Autodesk Inventor part; units mm, degrees
ref_plane "YZ Plane" through (0, 0, 0) normal (1, 0, 0) x (0, 1, 0)
ref_plane "XZ Plane" through (0, 0, 0) normal (0, 1, 0) x (-1, 0, 0)
ref_plane "XY Plane" through (0, 0, 0) normal (0, 0, 1) x (1, 0, 0)
sketch "Sketch1" plane through (0, 0, 0) normal (0, 1, 0) x (-1, 0, 0)
  arc A0 (0, -50) -> (0, 0) centre (-48.9898, -25) ccw
  arc A1 (0, -49) -> (0, -1) centre (-49.4874, -25) ccw
  line L0 (0, 0) -> (0, -50)
  line L1 (0, -12.5) -> (5.5721, -18.0721)
  line L2 (0, -12.5) -> (7.8802, -12.5) construction
  line L3 (0, -13.5) -> (5.704, -19.204)
  line L4 (0, -25) -> (5.7127, -30.7127)
  line L5 (0, -25) -> (8.079, -25) construction
  line L6 (0, -26) -> (5.6114, -31.6114)
  line L7 (0, -35) -> (4.157, -39.157)
  line L8 (0, -35) -> (5.8789, -35) construction
  line L9 (0, -36) -> (3.9417, -39.9417)
  arc A2 (0, 0) -> (0, -50) centre (48.9898, -25) ccw
  arc A3 (0, -1) -> (0, -49) centre (49.4874, -25) ccw
  line L10 (0, -12.5) -> (-5.5721, -18.0721)
  line L11 (0, -13.5) -> (-5.704, -19.204)
  line L12 (0, -25) -> (-5.7127, -30.7127)
  line L13 (0, -26) -> (-5.6114, -31.6114)
  line L14 (0, -35) -> (-4.157, -39.157)
  line L15 (0, -36) -> (-3.9417, -39.9417)
  line L16 (0.5, 0) -> (0.5, -50.0047)
  line L17 (-0.5, 0) -> (-0.5, -50.0047)
  point P0 (5.1659, -31.1659)
  point P1 (3.7628, -38.7628)
  point P2 (0.5, -35.5)
  point P3 (0.5, -26.5)
  point P4 (-3.7628, -38.7628)
  point P5 (-5.1659, -31.1659)
  point P6 (-0.5, -26.5)
  point P7 (-0.5, -35.5)
  point P8 (-5.2605, -30.2605)
  point P9 (-5.1441, -18.6441)
  point P10 (-0.5, -14)
  point P11 (-0.5, -25.5)
  point P12 (-4.9987, -17.4987)
  point P13 (-0.5, -2.0596)
  point P14 (-0.5, -13)
  point P15 (-0.5, -36.5)
  point P16 (-0.5, -47.9404)
  point P17 (-3.5525, -39.5525)
  point P18 (4.9987, -17.4987)
  point P19 (0.5, -13)
  point P20 (0.5, -2.0596)
  point P21 (3.5525, -39.5525)
  point P22 (0.5, -47.9404)
  point P23 (0.5, -36.5)
  point P24 (5.1441, -18.6441)
  point P25 (5.2605, -30.2605)
  point P26 (0.5, -25.5)
  point P27 (0.5, -14)
  dimension "d0" = 50
  dimension "d1" = 55
  dimension "d2" = 48
  dimension "d3" = 55
  dimension "d4" = 45
  dimension "d5" = 45
  dimension "d6" = 45
extrude "Extrusion1" add sketch "Sketch1" along normal blind 20 contours L9 A1 L7 A0 | A0 L16 A1 L9 | L7 A1 L6 A0 | A0 L0 A1 L16 | L9 L16 L7 A1 | L6 A1 L4 A0 | A2 L17 A3 L0 | A1 L0 L9 L16 | L9 L0 L7 L16 | L4 A1 L3 A0 | L6 L16 L4 A1 | L7 L0 L6 L16 | A3 L17 L15 L0 | A2 L15 A3 L17 | L15 L17 L14 L0 | L3 A1 L1 A0 | L6 L0 L4 L16 | L14 L17 L13 L0 | A2 L14 A3 L15 | L15 A3 L14 L17 | L1 A1 L16 A0 | L3 L16 L1 A1 | L4 L0 L3 L16 | L13 L17 L12 L0 | A2 L13 A3 L14 | L16 A1 L0 A0 | L3 L0 L1 L16 | L12 L17 L11 L0 | L13 A3 L12 L17 | A2 L12 A3 L13 | L0 A3 L17 A2 | L16 L1 L0 A1 | L11 L17 L10 L0 | A2 L11 A3 L12 | L0 L10 L17 A3 | L17 A3 L10 A2 | L11 A3 L10 L17 | A2 L10 A3 L11
sketch "Sketch2" plane through (0, 0, 0) normal (0, 0, 1) x (1, 0, 0)
  point P0 (0, 0)
sketch "Sketch3" plane through (0, 0, 0) normal (1, 0, 0) x (0, 1, 0)
  line L0 (0, 0) -> (20, 0)
  line L1 (0, -50) -> (20, -50)
  arc A0 (10, 0) -> (10, -50) centre (64.5436, -25) ccw
  arc A1 (11, 0) -> (11, -50) centre (65.5436, -25) ccw
  line L2 (11, 0) -> (11, -50) construction
  line L3 (11, 0) -> (61, 0) construction
  line L4 (11, 0) -> (20, 0)
  line L5 (20, -50) -> (20, 0)
  line L6 (20, 0) -> (20, -50)
  line L7 (20, -50) -> (11, -50)
  line L8 (10, 0) -> (0, 0)
  line L9 (0, 0) -> (0, -50)
  line L10 (10, -50) -> (0, -50)
  point P0 (11, 0)
  point P1 (11, -50)
  dimension "d9" = 60
  dimension "d10" = 50
  dimension "d11" = 90
  dimension "d12" = 60
extrude "Extrusion2" cut sketch "Sketch3" along normal mid plane 20 contours L0 A0 L1 L9 | L0 L5 L1 A1
Check sheet for the modelled part. Datum: model origin and axes. Units: mm. Give positions to 0.01 mm unless a question says otherwise; leave off trailing zeros. Order: outer loops, then holes, each group sorted by start corner. A loop starts at its lowest first (then second) coordinate and runs counter-clockwise, first axis right, second up. Notation, with made-up numbers: M 43.25,33 L 73.25,33 A25 ccw 73.25,68 Z; hole C -0.5,45 d11. An arc over 180 degrees is marked long. Answer as CSV lines item,"result". Start each with the question number.
Item 1: Cross-section at C-C on y = 7.75. Enter the section's corners in (x, z).
Item 2: Cross-section at B-B on x = -1.75. Enter the section's corners in (y, z).
Item 3: Thickness scan on line 1 (X direction, y = 6, z = -33.5); line 2 (Z direction, x = -0.75, y = 9.75); line 3 (Z direction, x = 3.5, y = 5.5). Record the ranges inside material, lowest first. Write a range as [from, to].
Item 4: Cross-section at D-D on x = -4.5. Enter the section's corners in (y, z).
Item 5: Gauge pin test, flat ends, axial feed: P1, Ø6, axis at x = -1.5, z = -38, coming from the +Y side; P2, Ø3.5, axis at y = 7.5, z = -40, coming from the -X side; P3, Ø4, axis at x = 0, z = -19, coming from the -Y side. Record the tip position at first contact, or that the pin passes through.
Item 6: Cross-section at A-A on z = -25. Enter the section's corners in (x, y).
Established:
1,outline,"M -3.59,-41.12 A55 ccw -2.49,-44.35 L -2,-44.35 A55 cw -3.1,-41.12 Z; M -3.59,-8.88 L -3.1,-8.88 A55 cw -2,-5.65 L -2.49,-5.65 A55 ccw Z; M -0.5,-44.35 L 0.5,-44.35 L 0.5,-41.12 L -0.5,-41.12 Z; M -0.5,-8.88 L 0.5,-8.88 L 0.5,-5.65 L -0.5,-5.65 Z; M 2,-44.35 L 2.49,-44.35 A55 ccw 3.59,-41.12 L 3.1,-41.12 A55 cw Z; M 2,-5.65 A55 cw 3.1,-8.88 L 3.59,-8.88 A55 ccw 2.49,-5.65 Z"
2,outline,"M 4.57,-26.75 A60 ccw 4.61,-27.75 L 5.61,-27.75 A60 cw 5.57,-26.75 Z; M 5.34,-15.25 L 6.34,-15.25 A60 cw 6.51,-14.25 L 5.51,-14.25 A60 ccw Z; M 5.71,-36.75 A60 ccw 5.91,-37.75 L 6.91,-37.75 A60 cw 6.71,-36.75 Z; M 7.97,-44.99 A60 ccw 8.42,-46.22 L 9.42,-46.22 A60 cw 8.97,-44.99 Z; M 7.97,-5.01 L 8.97,-5.01 A60 cw 9.42,-3.78 L 8.42,-3.78 A60 ccw Z"
3,line 1,"x = [-5.35, -4.85], [-0.5, 0.5], [4.85, 5.35]"
3,line 2,"z = [-48.47, -47.39], [-2.61, -1.53]"
3,line 3,"z = [-29.5, -28.5], [-17, -16]"
4,outline,"M 4.71,-29.5 A60 ccw 4.8,-30.5 L 5.8,-30.5 A60 cw 5.71,-29.5 Z; M 4.95,-18 L 5.95,-18 A60 cw 6.08,-17 L 5.08,-17 A60 ccw Z; M 5.47,-35.51 A60 ccw 5.92,-37.8 L 6.92,-37.8 A60 cw 6.47,-35.51 Z; M 5.47,-14.49 L 6.47,-14.49 A60 cw 6.92,-12.2 L 5.92,-12.2 A60 ccw Z"
5,P1,"stops at y = 7.67"
5,P2,"stops at x = -4.37"
5,P3,"stops at y = 4.68"
6,outline,"M -6.01,4.54 L -5.51,4.54 L -5.51,5.54 L -6.01,5.54 Z; M -0.5,4.54 L 0.5,4.54 L 0.5,5.54 L -0.5,5.54 Z; M 5.51,4.54 L 6.01,4.54 L 6.01,5.54 L 5.51,5.54 Z"
